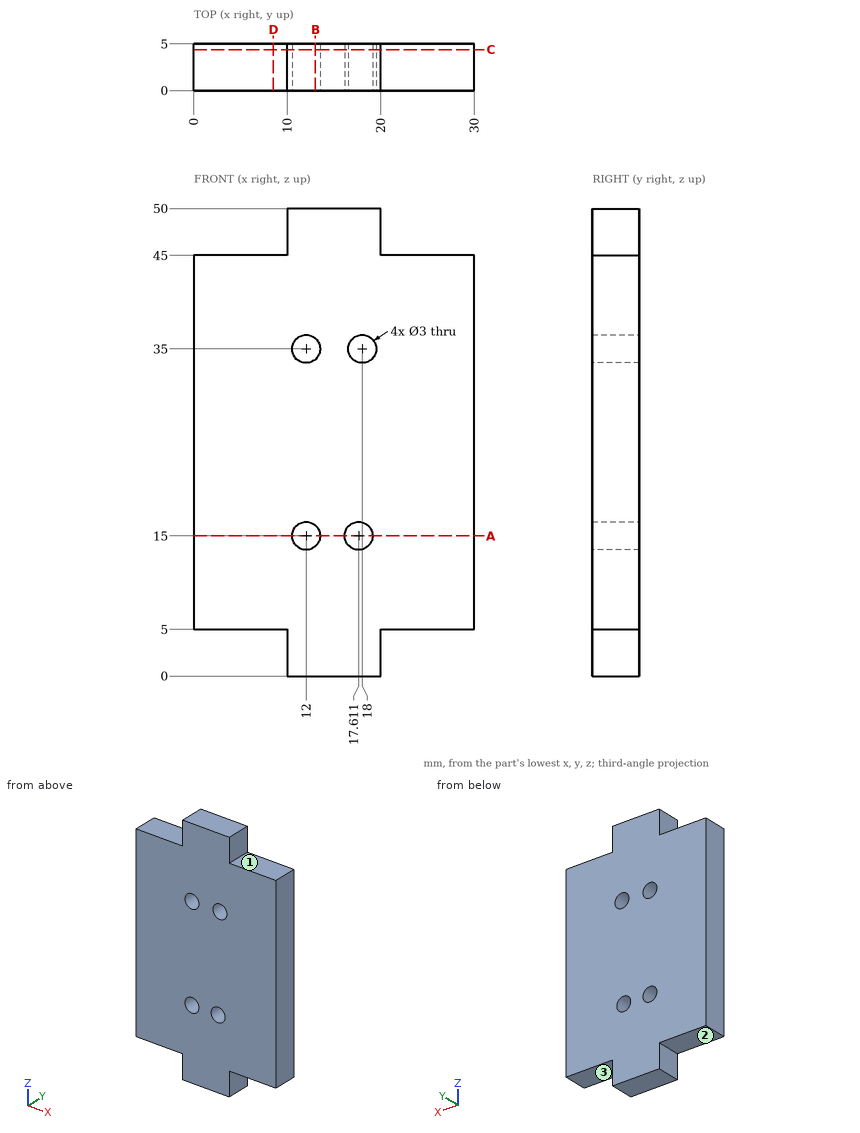
Answer from the drawing. Dimensions are ordinates in mm from the lowest x, y and z of the part. A direction names the side the tool comes from. Round coordinates to 2 decimals unless told otherwise and drop trailing zeros. Order: outer loops, then holes, each group sorted by start corner. A loop starts at its lowest first (then second) coordinate and runs counter-clockwise, first axis right, second up. Notation, with made-up numbers: (73, 59) -> (115, 59) arc R23 ccw to (115, 72) -> close; hole circle Ø9 at (73, -20). An arc over 180 degrees is marked (long way). Answer as CSV lines item,"result".
Q1. A cutting plane is placed at D-D on x = 8.5. Determine the outline of the cut face in (y, z).
Computed values:
outline,"(0, 5) -> (5, 5) -> (5, 45) -> (0, 45) -> close"
Q2. Given pin 1 (1.5 mm diameter, centred on x = 26, y = 1.5, fed in from +Z); pin 2 (8 mm diameter, centred on x = 24.5, z = 25, fed in from -Y); pin 3 (2.5 mm diameter, centred on x = 18, z = 35, fed in from +Y); pin 4 (1.5 mm diameter, centred on x = 3.5, y = 2.5, fed in from -Z), each flat-ended and moving along its own axis, determine where each tip first touches the part or whether it passes through.
Computed values:
pin 1,"stops at z = 45"
pin 2,"stops at y = 0"
pin 3,"passes through"
pin 4,"stops at z = 5"
Q3. A cutting plane is placed at C-C on y = 4.4. Determine the outline of the cut face in (x, z), plus the area to 3 significant figures.
Computed values:
outline,"(0, 5) -> (10, 5) -> (10, 0) -> (20, 0) -> (20, 5) -> (30, 5) -> (30, 45) -> (20, 45) -> (20, 50) -> (10, 50) -> (10, 45) -> (0, 45) -> close; hole circle Ø3 at (12, 15); hole circle Ø3 at (12, 35); hole circle Ø3 at (17.61, 15); hole circle Ø3 at (18, 35)"
area,"1,270 mm^2"
Q4. A cutting plane is placed at B-B on x = 13. Determine the outline of the cut face in (y, z), plus the area to 3 significant figures.
Computed values:
outline,"(0, 0) -> (5, 0) -> (5, 13.88) -> (0, 13.88) -> close; (0, 16.12) -> (5, 16.12) -> (5, 33.88) -> (0, 33.88) -> close; (0, 36.12) -> (5, 36.12) -> (5, 50) -> (0, 50) -> close"
area,"228 mm^2"
Q5. A cutting plane is placed at A-A on z = 15. Determine the outline of the cut face in (x, y).
Computed values:
outline,"(0, 0) -> (10.5, 0) -> (10.5, 5) -> (0, 5) -> close; (13.5, 0) -> (16.11, 0) -> (16.11, 5) -> (13.5, 5) -> close; (19.11, 0) -> (30, 0) -> (30, 5) -> (19.11, 5) -> close"
Q6. Which of the six approach directions +Z, -Z, +X, -X, +Y, -Y give full straight-line access (tool end or side, diameter ignored) to the marked faces 1, 2 and 3?
Computed values:
face 1,"+Z, +X, +Y, -Y"
face 2,"-Z, -X, +Y, -Y"
face 3,"-Z, +X, +Y, -Y"
Q7. Consider line 1 (X direction, y = 2.55, z = 35); line 2 (X direction, y = 3.1, z = 15); line 3 (Z direction, x = 12.5, y = 3.1) (1 decimal). Determine where each line is inside the solid, lowest interval first. Write a range as from..to.
Computed values:
line 1,"x = 0..10.5, 13.5..16.5, 19.5..30"
line 2,"x = 0..10.5, 13.5..16.11, 19.11..30"
line 3,"z = 0..13.6, 16.4..33.6, 36.4..50"
